CAD build for the part. Positions are in the model's coordinates, mm. Give positions to 0.01 mm unless a question says otherwise; leave off trailing zeros. Order: outer loops, then holes, each group sorted by start corner. A loop starts at its lowest first (then second) coordinate and runs counter-clockwise, first axis right, second up.
```python
from build123d import *

# Parameters (mm, degrees)
SKETCH1_W           = 276
SKETCH1_H           = 104.826000086
BOSS_EXTRUDE1_DEPTH = 6.35
CUT_EXTRUDE1_REACH  = 149.755
SKETCH2_R           = 2.2
CUT_EXTRUDE2_REACH  = 149.755
SKETCH3_R           = 2.2
CUT_EXTRUDE3_REACH  = 149.755
SKETCH4_R           = 7.9629
CUT_EXTRUDE4_REACH  = 149.755
SKETCH5_R           = 1.7


with BuildPart() as part:
    # Sketch1 → Boss-Extrude1 (new body)
    with BuildSketch(Plane(origin=(0, 0, 0), x_dir=(1, 0, 0), z_dir=(0, 1, 0))):
        Rectangle(SKETCH1_W, SKETCH1_H)
    extrude(amount=BOSS_EXTRUDE1_DEPTH)

    # Sketch2 → Cut-Extrude1 (cut, up to next)
    with BuildSketch(Plane(origin=(0, 6.35, 0), x_dir=(1, 0, 0), z_dir=(0, 1, 0)), mode=Mode.PRIVATE) as cut_extrude1_sk1:
        with Locations(Location((-130, 33.363000043, 0), (0, 0, 270))):
            Circle(SKETCH2_R)
    cut_extrude1_tool1 = extrude(cut_extrude1_sk1.sketch, amount=-CUT_EXTRUDE1_REACH, mode=Mode.PRIVATE) & part.part
    # Sketch2 → Cut-Extrude1 (cut, up to next)
    with BuildSketch(Plane(origin=(0, 6.35, 0), x_dir=(1, 0, 0), z_dir=(0, 1, 0)), mode=Mode.PRIVATE) as cut_extrude1_sk2:
        with Locations(Location((-130, -33.363000043, 0), (0, 0, 270))):
            Circle(SKETCH2_R)
    cut_extrude1_tool2 = extrude(cut_extrude1_sk2.sketch, amount=-CUT_EXTRUDE1_REACH, mode=Mode.PRIVATE) & part.part
    # Sketch2 → Cut-Extrude1 (cut, up to next)
    with BuildSketch(Plane(origin=(0, 6.35, 0), x_dir=(1, 0, 0), z_dir=(0, 1, 0)), mode=Mode.PRIVATE) as cut_extrude1_sk3:
        with Locations(Location((130, -33.363000043, 0), (0, 0, 270))):
            Circle(SKETCH2_R)
    cut_extrude1_tool3 = extrude(cut_extrude1_sk3.sketch, amount=-CUT_EXTRUDE1_REACH, mode=Mode.PRIVATE) & part.part
    # Sketch2 → Cut-Extrude1 (cut, up to next)
    with BuildSketch(Plane(origin=(0, 6.35, 0), x_dir=(1, 0, 0), z_dir=(0, 1, 0)), mode=Mode.PRIVATE) as cut_extrude1_sk4:
        with Locations(Location((130, 33.363000043, 0), (0, 0, 270))):
            Circle(SKETCH2_R)
    cut_extrude1_tool4 = extrude(cut_extrude1_sk4.sketch, amount=-CUT_EXTRUDE1_REACH, mode=Mode.PRIVATE) & part.part
    add(cut_extrude1_tool1.solids().sort_by_distance((-130, 6.35, -33.363))[0], mode=Mode.SUBTRACT)
    add(cut_extrude1_tool2.solids().sort_by_distance((-130, 6.35, 33.363))[0], mode=Mode.SUBTRACT)
    add(cut_extrude1_tool3.solids().sort_by_distance((130, 6.35, 33.363))[0], mode=Mode.SUBTRACT)
    add(cut_extrude1_tool4.solids().sort_by_distance((130, 6.35, -33.363))[0], mode=Mode.SUBTRACT)

    # Sketch3 → Cut-Extrude2 (cut, up to next)
    with BuildSketch(Plane(origin=(0, 6.35, 0), x_dir=(1, 0, 0), z_dir=(0, 1, 0)), mode=Mode.PRIVATE) as cut_extrude2_sk1:
        with Locations(Location((-106.885, 42.413000043, 0), (0, 0, 270))):
            Circle(SKETCH3_R)
    cut_extrude2_tool1 = extrude(cut_extrude2_sk1.sketch, amount=-CUT_EXTRUDE2_REACH, mode=Mode.PRIVATE) & part.part
    # Sketch3 → Cut-Extrude2 (cut, up to next)
    with BuildSketch(Plane(origin=(0, 6.35, 0), x_dir=(1, 0, 0), z_dir=(0, 1, 0)), mode=Mode.PRIVATE) as cut_extrude2_sk2:
        with Locations(Location((106.885, 42.413000043, 0), (0, 0, 270))):
            Circle(SKETCH3_R)
    cut_extrude2_tool2 = extrude(cut_extrude2_sk2.sketch, amount=-CUT_EXTRUDE2_REACH, mode=Mode.PRIVATE) & part.part
    add(cut_extrude2_tool1.solids().sort_by_distance((-106.885, 6.35, -42.413))[0], mode=Mode.SUBTRACT)
    add(cut_extrude2_tool2.solids().sort_by_distance((106.885, 6.35, -42.413))[0], mode=Mode.SUBTRACT)

    # Sketch4 → Cut-Extrude3 (cut, up to next)
    with BuildSketch(Plane(origin=(0, 6.35, 0), x_dir=(1, 0, 0), z_dir=(0, 1, 0)), mode=Mode.PRIVATE) as cut_extrude3_sk1:
        with Locations(Location((60, -16.543000155, 0), (0, 0, 270))):
            Circle(SKETCH4_R)
    cut_extrude3_tool1 = extrude(cut_extrude3_sk1.sketch, amount=-CUT_EXTRUDE3_REACH, mode=Mode.PRIVATE) & part.part
    add(cut_extrude3_tool1.solids().sort_by_distance((60, 6.35, 16.543))[0], mode=Mode.SUBTRACT)

    # Sketch5 → Cut-Extrude4 (cut, up to next)
    with BuildSketch(Plane(origin=(0, 6.35, 0), x_dir=(1, 0, 0), z_dir=(0, 1, 0)), mode=Mode.PRIVATE) as cut_extrude4_sk1:
        with Locations(Location((60, -3.843000155, 0), (0, 0, 270))):
            Circle(SKETCH5_R)
    cut_extrude4_tool1 = extrude(cut_extrude4_sk1.sketch, amount=-CUT_EXTRUDE4_REACH, mode=Mode.PRIVATE) & part.part
    # Sketch5 → Cut-Extrude4 (cut, up to next)
    with BuildSketch(Plane(origin=(0, 6.35, 0), x_dir=(1, 0, 0), z_dir=(0, 1, 0)), mode=Mode.PRIVATE) as cut_extrude4_sk2:
        with Locations(Location((72.7, -16.543000155, 0), (0, 0, 270))):
            Circle(SKETCH5_R)
    cut_extrude4_tool2 = extrude(cut_extrude4_sk2.sketch, amount=-CUT_EXTRUDE4_REACH, mode=Mode.PRIVATE) & part.part
    # Sketch5 → Cut-Extrude4 (cut, up to next)
    with BuildSketch(Plane(origin=(0, 6.35, 0), x_dir=(1, 0, 0), z_dir=(0, 1, 0)), mode=Mode.PRIVATE) as cut_extrude4_sk3:
        with Locations(Location((60, -29.243000155, 0), (0, 0, 270))):
            Circle(SKETCH5_R)
    cut_extrude4_tool3 = extrude(cut_extrude4_sk3.sketch, amount=-CUT_EXTRUDE4_REACH, mode=Mode.PRIVATE) & part.part
    # Sketch5 → Cut-Extrude4 (cut, up to next)
    with BuildSketch(Plane(origin=(0, 6.35, 0), x_dir=(1, 0, 0), z_dir=(0, 1, 0)), mode=Mode.PRIVATE) as cut_extrude4_sk4:
        with Locations(Location((47.3, -16.543000155, 0), (0, 0, 270))):
            Circle(SKETCH5_R)
    cut_extrude4_tool4 = extrude(cut_extrude4_sk4.sketch, amount=-CUT_EXTRUDE4_REACH, mode=Mode.PRIVATE) & part.part
    add(cut_extrude4_tool1.solids().sort_by_distance((60, 6.35, 3.843))[0], mode=Mode.SUBTRACT)
    add(cut_extrude4_tool2.solids().sort_by_distance((72.7, 6.35, 16.543))[0], mode=Mode.SUBTRACT)
    add(cut_extrude4_tool3.solids().sort_by_distance((60, 6.35, 29.243))[0], mode=Mode.SUBTRACT)
    add(cut_extrude4_tool4.solids().sort_by_distance((47.3, 6.35, 16.543))[0], mode=Mode.SUBTRACT)


solid = part.part
```
Item 1: Slice it at A-A (z = 12). Give the cut face in (x, y), and give its area (3 significant figures).
Item 2: Two-plate mould, pull along X, no slides. Class faces 1 (the face through (-138, 3, 1)), 2 (the face through (55.155, 3.219, 10.224)), 3 (the face through (-2, 6.35, -1)): released by +X, released by -X, zero draft, split by the parting line, or undercut.
Item 3: Wall check: L1, parallel to X at y = 5.25, z = -42.5; L2, parallel to Z at x = 130, y = 3; L3, parallel to X at y = 0.5, z = -34. Give the ranges that are in metal, low to high.
Item 4: Drop a flat-ended pin along its axis: pin 1 Ø4 at (x, z) = (-106.885, -42.413) entering from -Y. Give the stop position or say it passes through.
A:
1. outline: (-138, 0) - (53.46, 0) - (53.46, 6.35) - (-138, 6.35) - close; (66.54, 0) - (138, 0) - (138, 6.35) - (66.54, 6.35) - close
1. area: 1,670 mm2
2. face 1: released by -X
2. face 2: undercut
2. face 3: zero draft
3. L1: x = -138 to -109.08, -104.69 to 104.69, 109.08 to 138
3. L2: z = -52.41 to -35.56, -31.16 to 31.16, 35.56 to 52.41
3. L3: x = -138 to -132.11, -127.89 to 127.89, 132.11 to 138
4. pin 1: passes through
